Geometry: final body of the model. Coordinates: model frame, mm. A direction names the side the tool comes from. Give positions to 0.01 mm unless a question says otherwise; leave off trailing zeros. Write each loop counter-clockwise with the first axis right and the second up, starting at its lowest first coordinate (ties: lowest second). Pieces come first, ordered by that corner, then holes.
Q1. Pin query (flat end, axial travel): pin 1 Ø10.5 at (x, z) = (-145.923, 25.4) entering from -Y. Return the tip coordinate at first contact, or that it passes through.
Q2. Section B-B (z = 103). Return the cut outline in (x, y), plus the area to 3 significant figures.
Q3. Section A-A (z = 0). Return the cut outline in (x, y).
Q4. Reachability of faces 1 (the cylindrical face through (-98.94, 3.13, 119.99)), 2 (the flat face through (154.995, 3.219, 63.31)) from +Z, -Z, +X, -X, +Y, -Y: full face, straight path, thin tool, end or side. Return the list, or none.
Q5. Line query: line 1 (X direction, y = 5.25, z = 139.7); line 2 (X direction, y = 5.75, z = 55); line 3 (Z direction, x = -39.5, y = 1). Output: solid intervals per line, ascending.
Q6. Section C-C (y = 3.5). State how many separate pieces and enclosed holes the cut face has, plus the area to 3 significant figures.
Q7. Mould query, pull axis X, two halves, no side actions, for faces 3 (the flat face through (161.834, 3.131, 44.849)), 4 (the flat face through (130, 6.35, 33)), 5 (the cylindrical face through (124.923, 3.219, 69.074)). Classes: +X half, -X half, draft (parallel to the pull), parting line (faces both ways), or undercut.
Q8. Section D-D (z = -46). Return the cut outline in (x, y), plus the area to 3 significant figures.
from build123d import *

# Parameters (mm, degrees)
SKETCH1_R           = 3.2639
SKETCH1_R_2         = 133.223
SKETCH1_R_3         = 2.6289
SKETCH1_R_4         = 14.2875
BOSS_EXTRUDE1_DEPTH = 6.35
CUT_EXTRUDE1_DEPTH  = 6.35
FILLET1_R           = 6.35


with BuildPart() as part:
    # Sketch1 → Boss-Extrude1 (new body)
    with BuildSketch(Plane(origin=(0, 0, 0), x_dir=(1, 0, 0), z_dir=(0, 1, 0))):
        with BuildLine():
            Line((95.377, 152.4), (0, 152.4))
            ThreePointArc((0, 152.4), (-97.757028045, 120.848293921), (-158.623, 38.1))
            Line((-158.623, 38.1), (-158.623, -38.1))
            ThreePointArc((-158.623, -38.1), (-97.757028045, -120.848293921), (0, -152.4))
            Line((0, -152.4), (161.207253597, -152.4))
            ThreePointArc((161.207253597, -152.4), (171.540803487, -139.027863312), (173.54963847, -122.24808754))
            Line((173.54963847, -122.24808754), (149.785027389, 34.747190404))
            ThreePointArc((149.785027389, 34.747190404), (130.958683739, 97.447812085), (95.377, 152.4))
        make_face()
        with Locations(Location((108.077, -139.7, 0), (0, 0, 270))):
            Circle(SKETCH1_R, mode=Mode.SUBTRACT)
        with Locations(Location((-145.923, -25.4, 0), (0, 0, 270))):
            Circle(SKETCH1_R, mode=Mode.SUBTRACT)
        with Locations(Location((0, 0, 0), (0, 0, 270))):
            Circle(SKETCH1_R_2, mode=Mode.SUBTRACT)
        with Locations(Location((57.277, -139.7, 0), (0, 0, 270))):
            Circle(SKETCH1_R, mode=Mode.SUBTRACT)
        with Locations(Location((-145.923, 25.4, 0), (0, 0, 270))):
            Circle(SKETCH1_R, mode=Mode.SUBTRACT)
        with Locations(Location((57.277, 139.7, 0), (0, 0, 270))):
            Circle(SKETCH1_R, mode=Mode.SUBTRACT)
        with Locations(Location((166.516908963, -119.805057995, 0), (0, 0, 270))):
            Circle(SKETCH1_R_3, mode=Mode.SUBTRACT)
        with Locations(Location((117.797598231, -134.194942005, 0), (0, 0, 270))):
            Circle(SKETCH1_R_3, mode=Mode.SUBTRACT)
        with Locations(Location((142.157253597, -127, 0), (0, 0, 270))):
            Circle(SKETCH1_R_4, mode=Mode.SUBTRACT)
    extrude(amount=BOSS_EXTRUDE1_DEPTH)

    # Sketch2 → Cut-Extrude1 (cut)
    with BuildSketch(Plane(origin=(0, 6.35, 0), x_dir=(1, 0, 0), z_dir=(0, 1, 0))):
        with BuildLine():
            Line((81.096337026, -117.475), (159.907199476, -95.764025273))
            Line((159.907199476, -95.764025273), (142.748, 17.594164432))
            Line((142.748, 17.594164432), (142.748, 0))
            ThreePointArc((142.748, 0), (126.398835876, -66.33495152), (81.096337026, -117.475))
        make_face()
    extrude(amount=-CUT_EXTRUDE1_DEPTH, mode=Mode.SUBTRACT)

    # Fillet1
    fillet1_edges = [part.edges().sort_by_distance(p)[0] for p in [
        (81.096337026, 3.175, 117.475),
        (142.748, 3.175, -17.594164432),
        (159.907199476, 3.175, 95.764025273),
    ]]
    fillet(fillet1_edges, radius=FILLET1_R)


solid = part.part
Computed:
1. pin 1: stops at y = 0
2. outline: (-118.66, 0) - (-84.49, 0) - (-84.49, 6.35) - (-118.66, 6.35) - close; (84.49, 0) - (100.8, 0) - (100.8, 6.35) - (84.49, 6.35) - close; (133.64, 0) - (170.64, 0) - (170.64, 6.35) - (133.64, 6.35) - close
2. area: 555 mm2
3. outline: (-158.62, 0) - (-133.22, 0) - (-133.22, 6.35) - (-158.62, 6.35) - close; (133.22, 0) - (155.04, 0) - (155.04, 6.35) - (133.22, 6.35) - close
4. face 1: +Z, -X, +Y, -Y
4. face 2: +Y, -Y
5. line 1: x = -63.92 to 54.01, 60.54 to 104.81, 111.34 to 135.61, 148.7 to 171.26
5. line 2: x = -151.94 to -121.34, 121.34 to 131.73, 153.74 to 163.37
5. line 3: z = -147.67 to -127.23, 127.23 to 147.67
6. separate pieces: 1
6. enclosed holes: 10
6. area: 25,400 mm2
7. face 3: +X half
7. face 4: draft
7. face 5: undercut
8. outline: (-155.77, 0) - (-125.03, 0) - (-125.03, 6.35) - (-155.77, 6.35) - close; (125.03, 0) - (147.8, 0) - (147.8, 6.35) - (125.03, 6.35) - close
8. area: 340 mm2
